Can you work these out from the model? Positions are in its coordinate system, mm. Face numbers are marked on the shaded views. A direction names the side the tool comes from. Round coordinates to 2 decimals unless told otherwise and drop trailing zeros. Write each loop counter-clockwise with the first axis right and the second up, starting at its lowest first coordinate (ties: lowest second). Pieces come first, ordered by that corner, then holes. Notation, with made-up numbers: M 18,23.25 L 28,23.25 A17 ccw 28,30.25 Z; hole C 10,-35.5 d4. An arc over 180 degrees is marked long. Answer in a Markdown table with one row per item. Add a question column.
(1) If I drill on probe 1 along Y at (x, z) = (8.5, 77); probe 2 along Z at (x, y) = (28, 4.25); probe 3 along Z at (x, y) = (29, 17), over which ranges is the centre line in solid material (lowest first)?
(2) Suppose I cut it at C-C, the plane x = 35.5. Write out the boundary of the cut face in (y, z), then the cut area to 3 significant figures.
(3) For the marked faces 1, 2, 3, 4 and 5, which set-ups out of +Z, -Z, +X, -X, +Y, -Y let a thin tool reach every point of the face, with its end or its side?
(4) I'm going to push flat-ended pins straight in: pin 1 (1.5 mm diameter, centred on x = 4, y = -14.5, fed in from +Z); pin 2 (1.5 mm diameter, centred on y = 10.5, z = 13.5, fed in from -X); pin 3 (5 mm diameter, centred on x = 29.5, z = 97, fed in from -Y); pin 4 (9 mm diameter, centred on x = 29.5, z = 97, fed in from +Y). Where does each tip first touch, or does it pass through?
(5) Suppose I cut it at A-A, the plane y = -9. Write out the boundary of the cut face in (x, z).
(6) Suppose I cut it at D-D, the plane z = 97. Write out the boundary of the cut face in (x, y), then the cut area to 3 significant figures.
(7) Suppose I cut it at B-B, the plane x = 21. Write out the boundary of the cut face in (y, z).
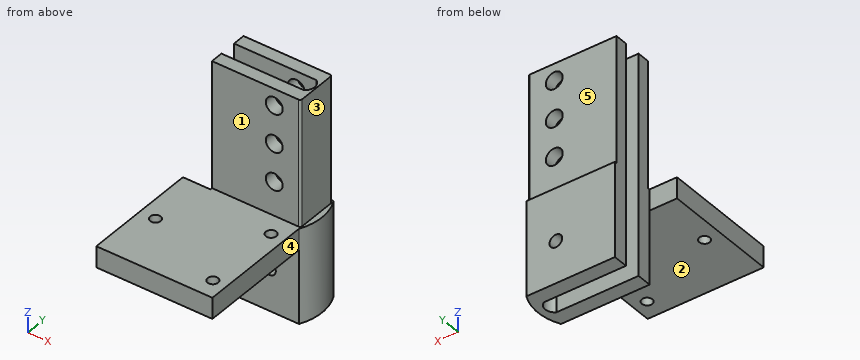
from build123d import *

# Parameters (mm, degrees)
PAD_DEPTH       = 45
SKETCH001_W     = 55
SKETCH001_H     = 10
PAD001_DEPTH    = 55
SKETCH002_R     = 3
POCKET_DEPTH    = 22
SKETCH003_R     = 2.5
POCKET001_DEPTH = 10
PAD002_DEPTH    = 60
SKETCH005_R     = 4
POCKET002_DEPTH = 20


with BuildPart() as part:
    # Sketch → Pad (new body)
    with BuildSketch(Plane.XY):
        with BuildLine():
            Line((0, 22), (42, 22))
            ThreePointArc((42, 0), (44.669271, 11), (42, 22))
            Line((42, 0), (0, 0))
            Line((0, 7), (0, 0))
            Line((38.9, 7), (0, 7))
            ThreePointArc((38.9, 7), (41.228437, 11), (38.9, 15))
            Line((0, 15), (38.9, 15))
            Line((0, 22), (0, 15))
        make_face()
    extrude(amount=PAD_DEPTH)

    # Sketch001 (on Face4 of Pad) → Pad001 (join)
    with BuildSketch(Plane.XZ):
        with Locations((14.5, 40)):
            Rectangle(SKETCH001_W, SKETCH001_H)
    extrude(amount=PAD001_DEPTH)

    # Sketch002 (on Face8 of Pad001) → Pocket (cut)
    with BuildSketch(Plane.XZ):
        with Locations((28, 20)):
            Circle(SKETCH002_R)
    extrude(amount=-POCKET_DEPTH, mode=Mode.SUBTRACT)

    # Sketch003 (on Face12 of Pocket) → Pocket001 (cut)
    with BuildSketch(Plane.XY.offset(45)):
        with Locations((35.5, -9)):
            Circle(SKETCH003_R)
        with Locations((35.5, -46)):
            Circle(SKETCH003_R)
        with Locations((-5.5, -27.5)):
            Circle(SKETCH003_R)
    extrude(amount=-POCKET001_DEPTH, mode=Mode.SUBTRACT)

    # Sketch004 (on Face5 of Pocket001) → Pad002 (join)
    with BuildSketch(Plane.XY.offset(45)):
        with BuildLine():
            Line((0, 21), (41, 21))
            ThreePointArc((42, 20), (41.707107, 20.707107), (41, 21))
            Line((42, 20), (42, 2))
            ThreePointArc((41, 1), (41.707107, 1.292893), (42, 2))
            Line((41, 1), (0, 1))
            Line((0, 1), (0, 7))
            Line((0, 7), (39, 7))
            ThreePointArc((39, 7), (41.232207, 11), (39, 15))
            Line((39, 15), (0, 15))
            Line((0, 15), (0, 21))
        make_face()
    extrude(amount=PAD002_DEPTH)

    # Sketch005 → Pocket002 (cut)
    with BuildSketch(Plane.XZ.offset(-1)):
        with Locations((29.5, 61)):
            Circle(SKETCH005_R)
        with Locations((29.5, 79)):
            Circle(SKETCH005_R)
        with Locations((29.5, 97)):
            Circle(SKETCH005_R)
    extrude(amount=-POCKET002_DEPTH, mode=Mode.SUBTRACT)


solid = part.part
Calculated:
| question | item | result |
|---|---|---|
| 1 | probe 1 | 1 to 7, 15 to 21 |
| 1 | probe 2 | 0 to 17, 23 to 57.29, 64.71 to 75.29, 82.71 to 93.29, 100.71 to 105 |
| 1 | probe 3 | 0 to 17.17, 22.83 to 57.03, 64.97 to 75.03, 82.97 to 93.03, 100.97 to 105 |
| 2 | outline | M -55,35 L -48.5,35 L -48.5,45 L -55,45 Z; M -43.5,35 L -11.5,35 L -11.5,45 L -43.5,45 Z; M -6.5,35 L 0,35 L 0,0 L 7,0 L 7,105 L 1,105 L 1,45 L -6.5,45 Z; M 15,0 L 22,0 L 22,45 L 21,45 L 21,105 L 15,105 Z |
| 2 | area | 1,800 mm² |
| 3 | face 1 | +Z, +X, -X, -Y |
| 3 | face 2 | -Z, +X, -X, -Y |
| 3 | face 3 | +Z, +X, +Y, -Y |
| 3 | face 4 | +Z, -Z, +X, -Y |
| 3 | face 5 | +Z, +X, -X, +Y |
| 4 | pin 1 | z = 45 |
| 4 | pin 2 | x = 41.06 |
| 4 | pin 3 | through |
| 4 | pin 4 | y = 21 |
| 5 | outline | M -13,35 L 33,35 L 33,45 L -13,45 Z; M 38,35 L 42,35 L 42,45 L 38,45 Z |
| 6 | outline | M 0,1 L 25.5,1 L 25.5,7 L 0,7 Z; M 0,15 L 25.5,15 L 25.5,21 L 0,21 Z; M 33.5,1 L 41,1 A1 ccw 42,2 L 42,20 A1 ccw 41,21 L 33.5,21 L 33.5,15 L 39,15 A4.7 cw 39,7 L 33.5,7 Z |
| 6 | area | 419 mm² |
| 7 | outline | M -55,35 L 0,35 L 0,0 L 7,0 L 7,105 L 1,105 L 1,45 L -55,45 Z; M 15,0 L 22,0 L 22,45 L 21,45 L 21,105 L 15,105 Z |
